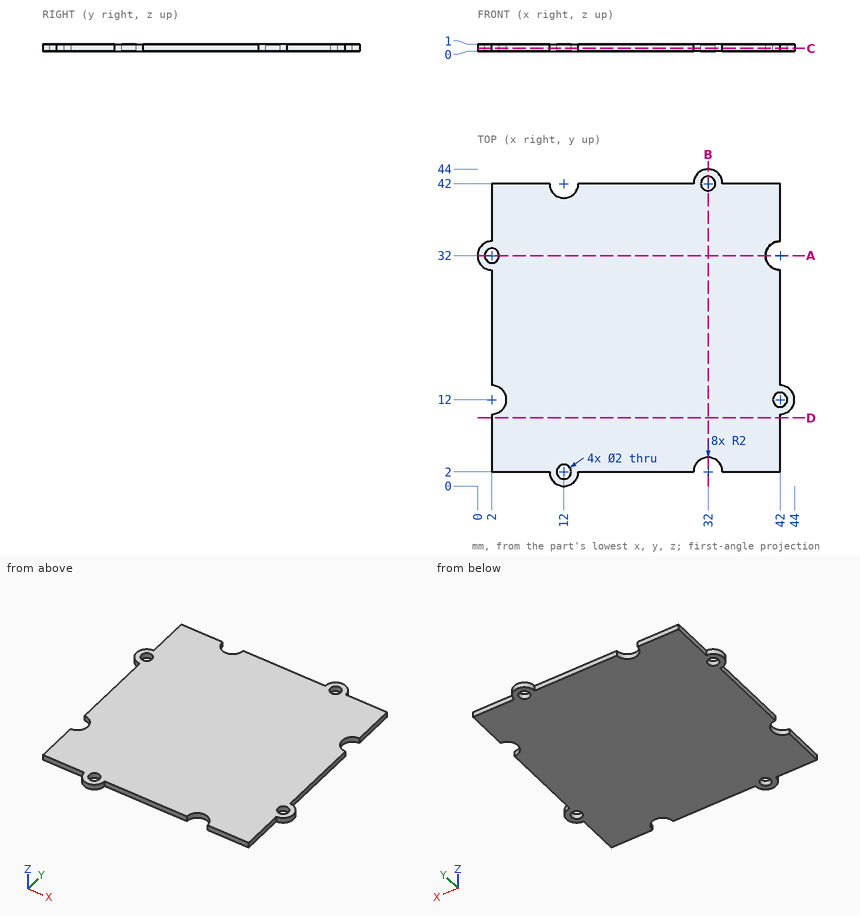
Source: three-view drawing plus pictorial views. Frame: mm from the lowest corner of the part. Round coordinates to 2 decimals unless told otherwise and drop trailing zeros. Order: outer loops, then holes, each group sorted by start corner. A loop starts at its lowest first (then second) coordinate and runs counter-clockwise, first axis right, second up. Notation, with made-up numbers: M 66,25.5 L 101,25.5 A12 ccw 101,39.5 Z; hole C -9,53 d7. An arc over 180 degrees is marked long. One line per item, written item: value.
(1) Cut plane B-B (x = 32). Return the cut outline in (y, z).
Result sheet:
outline: M 4,0 L 41,0 L 41,1 L 4,1 Z; M 43,0 L 44,0 L 44,1 L 43,1 Z
(2) Cut plane D-D (y = 9.5). Return the cut outline in (x, z).
Result sheet:
outline: M 2,0 L 42,0 L 42,1 L 2,1 Z
(3) Cut plane C-C (z = 0.4). Return the cut outline in (x, y).
Result sheet:
outline: M 2,2 L 10,2 A2 ccw 14,2 L 30,2 A2 cw 34,2 L 42,2 L 42,10 A2 ccw 42,14 L 42,30 A2 cw 42,34 L 42,42 L 34,42 A2 ccw 30,42 L 14,42 A2 cw 10,42 L 2,42 L 2,34 A2 ccw 2,30 L 2,14 A2 cw 2,10 Z; hole C 2,32 d2; hole C 12,2 d2; hole C 32,42 d2; hole C 42,12 d2
(4) Cut plane A-A (y = 32). Return the cut outline in (x, z), and give its area (3 significant figures).
Result sheet:
outline: M 0,0 L 1,0 L 1,1 L 0,1 Z; M 3,0 L 40,0 L 40,1 L 3,1 Z
area: 38.0 mm2
(5) Line query: probe 1 along Y at (x, z) = (32, 0.5); probe 2 along Y at (x, z) = (12, 0.65). Output: solid intervals per line, ascending. Write a range as [from, to].
Result sheet:
probe 1: [4, 41], [43, 44]
probe 2: [0, 1], [3, 40]
